```python
from build123d import *

# Parameters (mm, degrees)
SKETCH5_R           = 1.6
BOSS_EXTRUDE2_DEPTH = 2
SKETCH6_R           = 6
BOSS_EXTRUDE3_DEPTH = 15
FILLET1_R           = 1
BOSS_EXTRUDE5_DEPTH = 0.6


with BuildPart() as part:
    # Sketch5 → Boss-Extrude2 (new body)
    with BuildSketch(Plane(origin=(0, 0, 0), x_dir=(1, 0, 0), z_dir=(0, 1, 0))):
        with BuildLine():
            Line((-11.250000051, -22.142785594), (-3.22490315, -22.142785594))
            ThreePointArc((-3.22490315, -22.142785594), (-5.1e-08, -27.342785594), (3.224903048, -22.142785594))
            Line((3.224903048, -22.142785594), (11.249999949, -22.142785594))
            ThreePointArc((11.249999949, -22.142785594), (24.240381006, -14.642785594), (24.240381006, 0.357214406))
            Line((24.240381006, 0.357214406), (20.227832555, 7.30715219))
            ThreePointArc((20.227832555, 7.30715219), (23.118713105, 12.700000199), (17.002929456, 12.892848208))
            Line((17.002929456, 12.892848208), (12.990381006, 19.842785992))
            ThreePointArc((12.990381006, 19.842785992), (-5.1e-08, 27.342785992), (-12.990381108, 19.842785992))
            Line((-12.990381108, 19.842785992), (-17.002929558, 12.892848208))
            ThreePointArc((-17.002929558, 12.892848208), (-23.118713208, 12.700000199), (-20.227832658, 7.30715219))
            Line((-20.227832658, 7.30715219), (-24.240381108, 0.357214406))
            ThreePointArc((-24.240381108, 0.357214406), (-24.240381108, -14.642785594), (-11.250000051, -22.142785594))
        make_face()
        with Locations((20.001021652, 10.900000199)):
            Circle(SKETCH5_R, mode=Mode.SUBTRACT)
        with Locations((-5.1e-08, -23.742785594)):
            Circle(SKETCH5_R, mode=Mode.SUBTRACT)
        with Locations((-20.001021754, 10.900000199)):
            Circle(SKETCH5_R, mode=Mode.SUBTRACT)
    extrude(amount=BOSS_EXTRUDE2_DEPTH)

    # Sketch6 → Boss-Extrude3 (add)
    with BuildSketch(Plane(origin=(0, 0, 0), x_dir=(1, 0, 0), z_dir=(0, 1, 0))):
        with Locations((-0.060025126, 12.462836141)):
            Circle(SKETCH6_R)
        with Locations((11.189974874, -7.022735444)):
            Circle(SKETCH6_R)
        with Locations((-11.310025126, -7.022735444)):
            Circle(SKETCH6_R)
    extrude(amount=BOSS_EXTRUDE3_DEPTH)

    # Fillet1
    fillet1_edges = [part.edges().sort_by_distance(p)[0] for p in [
        (-6.060025126, 15, -12.462836141),
        (5.189974874, 15, 7.022735444),
        (-17.310025126, 15, 7.022735444),
    ]]
    fillet(fillet1_edges, radius=FILLET1_R)

    # Sketch7 → Boss-Extrude5 (add)
    with BuildSketch(Plane(origin=(18.334964129, 0, -10.585696476), x_dir=(-0.5, 0, -0.866025404), z_dir=(0.866025404, 0, -0.5))):
        with BuildLine():
            ThreePointArc((-10.342014969, 1.052839651), (-11.339215101, 1), (-10.342014969, 0.947160349))
            ThreePointArc((-10.342014969, 0.947160349), (-9.94912129, 1), (-10.342014969, 1.052839651))
        make_face()
    extrude(amount=BOSS_EXTRUDE5_DEPTH)


solid = part.part
```
The model under review builds one solid part; all positions refer to its coordinate system, in mm. A direction names the side the tool comes from. Coordinates: 2 decimals unless noted, no trailing zeros. Write each loop counter-clockwise with the first axis right and the second up, starting at its lowest first coordinate (ties: lowest second). Pieces come first, ordered by that corner, then holes. Notation, with made-up numbers: (82.5, 15.5) -> (124.5, 15.5) arc R25 ccw to (124.5, 30.5) -> close; hole circle Ø4 at (70.5, 88.5). An arc over 180 degrees is marked (long way). One line per item, written item: value. Start each with the question number.
Q1. Add section C-C, the plane z = 21. Give the boundary of the cut face in (x, y), then the cut area to 3 significant figures.
Q2. Add section B-B, the plane y = 4.5. Give the boundary of the cut face in (x, z), then the cut area to 3 significant figures.
Q3. The part is to be moulded in two halves that separate along Z. For faces 1 (the face through (22.262, 0.986, -3.784)), 2 (the face through (0, 15, -13)), 3 (the face through (-14.969, 0.986, -16.416)), say which applies: +Z half, -Z half, draft (parallel to the pull), parting line (faces both ways), or undercut.
Q4. Add section D-D, the plane z = -3. Give the boundary of the cut face in (x, y), then the cut area to 3 significant figures.
Q5. For faces 4 (the face through (0, 2, 0)), 5 (the face through (11, 15, 7)), 6 (the face through (15.025, 0.986, -16.319)), 7 (the face through (-22.206, 0.986, -3.881)), list the 3-axis set-ups (+Z, -Z, +X, -X, +Y, -Y) from which the entire face can be reached by the end or side of a thin tool; tool diameter is ignored.
Q6. To check wall thickness, follow probe 1 along X at (y, z) = (0.4, -10.9); probe 2 along Y at (x, z) = (6, 1.5); probe 3 along Z at (x, y) = (0, 0.7). State the ranges of each line that lie inside material, in increasing order.
Q7. Add section A-A, the plane z = -10.9. Count the separate pieces of the cut face and the enclosed holes in it, then the cut area to 3 significant figures.
Q8. Clearance check with flat-ended pins moving along their axes: P1, Ø1, axis at y = 12, z = -10.5, coming from the +X side; P2, Ø8, axis at x = -7.5, y = 3.5, coming from the -Z side; P3, Ø5, axis at x = -13, y = 10.5, coming from the +Z side; P4, Ø1.9, axis at x = 0, z = 23.74, coming from the -Y side. State where each tip first meets the part, or that it passes through.
Response:
1. outline: (-16.99, 0) -> (16.99, 0) -> (16.99, 2) -> (-16.99, 2) -> close
1. area: 68.0 mm²
2. outline: circle Ø12 at (-11.31, 7.02); circle Ø12 at (-0.06, -12.46); circle Ø12 at (11.19, 7.02)
2. area: 339 mm²
3. face 1: undercut
3. face 2: draft
3. face 3: -Z half
4. outline: (-22.71, 0) -> (22.71, 0) -> (22.71, 2) -> (-22.71, 2) -> close
4. area: 90.9 mm²
5. face 4: +Y
5. face 5: +Z, -Z, +X, -X, +Y
5. face 6: -Z, +Y, -Y
5. face 7: -X, +Y, -Y
6. probe 1: -23.6 to -21.6, -18.4 to 18.4, 21.6 to 23.6
6. probe 2: 0 to 2
6. probe 3: -27.34 to 22.14, 25.34 to 27.34
7. separate pieces: 3
7. enclosed holes: 0
7. area: 232 mm²
8. P1: x = 5.76
8. P2: z = -26.86
8. P3: z = 13.02
8. P4: through
